Check sheet for the modelled part. Datum: model origin and axes. Units: mm. Coordinates: 2 decimals unless noted, no trailing zeros. Order: outer loops, then holes, each group sorted by start corner. A loop starts at its lowest first (then second) coordinate and runs counter-clockwise, first axis right, second up.
Autodesk Fusion 360 part; units mm, degrees
sketch "Sketch1" plane through (0, 0, 0) normal (0, 0, 1) x (1, 0, 0) in component "base_layer"
  line L0 (0, 0) -> (113, 0)
  line L1 (113, 0) -> (113, 63)
  line L2 (113, 63) -> (0, 63)
  line L3 (0, 63) -> (0, 0)
  line L4 (9, 58) -> (12, 58)
  line L5 (104, 58) -> (101, 58)
  line L6 (13, 58) -> (14, 58)
  line L7 (15, 57) -> (15, 6)
  line L8 (14, 5) -> (13, 5)
  line L9 (12, 6) -> (12, 57)
  line L10 (100, 58) -> (99, 58)
  line L11 (98, 57) -> (98, 6)
  line L12 (99, 5) -> (100, 5)
  line L13 (101, 6) -> (101, 57)
  arc A0 (13, 58) -> (12, 57) centre (13, 57) ccw
  arc A1 (15, 57) -> (14, 58) centre (14, 57) ccw
  arc A2 (12, 6) -> (13, 5) centre (13, 6) ccw
  arc A3 (14, 5) -> (15, 6) centre (14, 6) ccw
  arc A4 (99, 58) -> (98, 57) centre (99, 57) ccw
  arc A5 (101, 57) -> (100, 58) centre (100, 57) ccw
  arc A6 (100, 5) -> (101, 6) centre (100, 6) ccw
  arc A7 (98, 6) -> (99, 5) centre (99, 6) ccw
  circle A8 centre (25, 50) radius 5
  circle A9 centre (25, 50) radius 5
  circle A10 centre (55.5469, 49.9659) radius 5
  circle A11 centre (71.1094, 50.2422) radius 5
  circle A12 centre (71.3194, 50.1842) radius 5
  circle A13 centre (86.6177, 49.7772) radius 5
  circle A14 centre (25, 50) radius 5
  circle A15 centre (24, 32) radius 5
  circle A16 centre (23.9972, 13.23) radius 5
  circle A17 centre (41.6022, 32.5064) radius 5
  circle A18 centre (41.1565, 13.5642) radius 5
  circle A19 centre (39.708, 50.3343) radius 5
  circle A20 centre (57.7588, 33.1749) radius 5
  circle A21 centre (73, 33) radius 5
  circle A22 centre (88.5119, 34.4006) radius 5
  circle A23 centre (58.4273, 14.0099) radius 5
  circle A24 centre (74.8067, 14.4556) radius 5
  circle A25 centre (88.9576, 14.6785) radius 5
  point P0 (15, 58)
  point P1 (15, 5)
  point P2 (98, 58)
  dimension "d1" = 113
  dimension "d2" = 63
  dimension "d5" = 5
  dimension "d7" = 5
  dimension "d14" = 3
  dimension "d15" = 5
  dimension "d16" = 3
  dimension "d17" = 5
  dimension "d18" = 1
  dimension "d19" = 1
  dimension "d20" = 1
  dimension "d21" = 1
  dimension "d22" = 10
  dimension "d23" = 10
  dimension "d24" = 10
  dimension "d25" = 10
  dimension "d26" = 10
  dimension "d27" = 10
  dimension "d28" = 10
  dimension "d29" = 10
  dimension "d30" = 10
  dimension "d31" = 10
  dimension "d32" = 10
  dimension "d33" = 10
  dimension "d34" = 10
  dimension "d35" = 10
  dimension "d36" = 10
  dimension "d37" = 10
  dimension "d38" = 10
  dimension "d39" = 10
extrude "Extrude1" add sketch "Sketch1" along normal blind 2 in component "base_layer"
fillet "Fillet1" radius 1 4 edges at (113, 31.5, 2) (56.5, 63, 2) (0, 31.5, 2) (56.5, 0, 2) in component "base_layer"
component "base_layer" placed x (1, 0, 0) y (0, 1, 0) z (0, 0, 1) at (0, 0, 0)
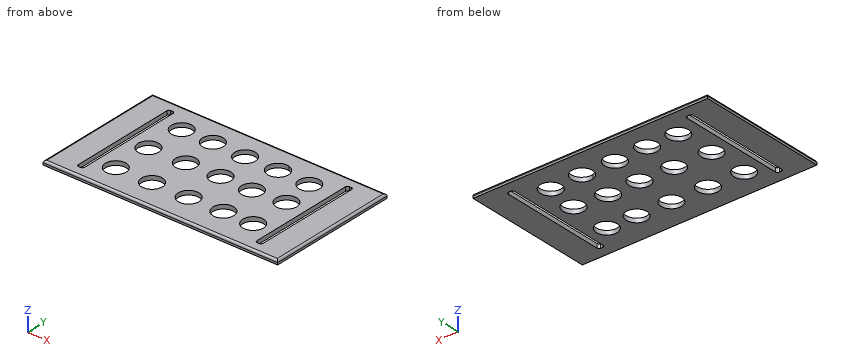
(1) Thickness scan on probe 1 along X at (y, z) = (56, 1); probe 2 along X at (y, z) = (23, 1.65); probe 3 along Y at (x, z) = (24, 1.55). Record the ranges inside material, lowest first.
Filled in:
probe 1: x = 0 to 12, 15 to 98, 101 to 113
probe 2: x = 0.24 to 12, 15 to 98, 101 to 112.76
probe 3: y = 0.16 to 8.23, 18.23 to 27, 37 to 45.1, 54.9 to 62.84
(2) Cross-section at D-D (x = 89.5). Enter the section's corners in (y, z), and give its area (3 significant figures).
Filled in:
outline: (0, 0) - (9.71, 0) - (9.71, 2) - (1, 2) arc R1 ccw to (0, 1) - close; (19.65, 0) - (29.5, 0) - (29.5, 2) - (19.65, 2) - close; (39.3, 0) - (45.69, 0) - (45.69, 2) - (39.3, 2) - close; (53.86, 0) - (63, 0) - (63, 1) arc R1 ccw to (62, 2) - (53.86, 2) - close
area: 69.7 mm2
(3) Cross-section at B-B (y = 46.5). Count the separate pieces of the cut face and the enclosed holes in it, and give its area (3 significant figures).
Filled in:
separate pieces: 8
enclosed holes: 0
area: 143 mm2
(4) Go/stop test with flat-tipped pins: P1, Ø16, axis at x = 74.81, y = 14.46, coming from the -Z side; P2, Ø6, axis at x = 88.96, y = 14.68, coming from the -Z side. Record where each tip stops, or that it passes through.
Filled in:
P1: stops at z = 0
P2: passes through
(5) Cross-section at A-A (x = 24). Enter the section's corners in (y, z), and give its area (3 significant figures).
Filled in:
outline: (0, 0) - (8.23, 0) - (8.23, 2) - (1, 2) arc R1 ccw to (0, 1) - close; (18.23, 0) - (27, 0) - (27, 2) - (18.23, 2) - close; (37, 0) - (45.1, 0) - (45.1, 2) - (37, 2) - close; (54.9, 0) - (63, 0) - (63, 1) arc R1 ccw to (62, 2) - (54.9, 2) - close
area: 66.0 mm2
